from build123d import *

# Parameters (mm, degrees)
F0_W     = 72.5
F0_H     = 50
F1_DEPTH = 3
F2_R     = 5
F4_DEPTH = 8
F5_R     = 3
F7_DEPTH = 33
F8_R     = 2


with BuildPart() as f1:
    # F0 (on Top) → F1 (new body)
    with BuildSketch(Plane.XY):
        Rectangle(F0_W, F0_H)
    extrude(amount=F1_DEPTH)

    # F2
    f2_edges = [f1.edges().sort_by_distance(p)[0] for p in [
        (36.25, -25, 1.5),
        (-36.25, -25, 1.5),
    ]]
    fillet(f2_edges, radius=F2_R)

    # F3 (on face) → F4 (join)
    with BuildSketch(Plane(origin=(0, 25, 0), x_dir=(-1, 0, 0), z_dir=(0, 1, 0))):
        with BuildLine():
            Line((36.25, 3), (36.25, 8.712942712))
            ThreePointArc((36.25, 8.712942712), (0, 11.712942712), (-36.25, 8.712942712))
            Line((-36.25, 8.712942712), (-36.25, 3))
            Line((-36.25, 3), (36.25, 3))
        make_face()
    extrude(amount=-F4_DEPTH)

    # F5
    f5_edges = [f1.edges().sort_by_distance(p)[0] for p in [
        (36.25, 21, 8.712943),
        (-36.25, 21, 8.712943),
    ]]
    fillet(f5_edges, radius=F5_R)

    # F6 (on face) → F7 (join)
    with BuildSketch(Plane.XZ.offset(-17)):
        with BuildLine():
            Line((32.25, 3), (36.25, 3))
            Line((36.25, 3), (36.25, 6.1565184682))
            ThreePointArc((36.25, 6.1565184682), (35.527695785, 8.1089789443), (33.7085987261, 9.1212591328))
            ThreePointArc((33.7085987261, 9.1212591328), (32.9794838617, 9.2327934458), (32.25, 9.3418882854))
            Line((32.25, 9.3418882854), (32.25, 3))
        make_face()
    extrude(amount=F7_DEPTH)

    # F8
    f8_edges = [f1.edges().sort_by_distance(p)[0] for p in [
        (36.25, -16, 4.578259),
    ]]
    fillet(f8_edges, radius=F8_R)

    # F9: F1 across plane


with BuildPart() as f1_1:
    add(f1.part)
    add(f1.part.mirror(Plane.YZ))


solid = f1_1.part
Source: CAD feature listing. Evaluate the final solid. Frame: model axes, mm. A direction names the side the tool comes from. Round coordinates to 2 decimals unless told otherwise and drop trailing zeros. Write each loop counter-clockwise with the first axis right and the second up, starting at its lowest first coordinate (ties: lowest second). Pieces come first, ordered by that corner, then holes. Notation, with made-up numbers: (49, 53.5) - (77, 53.5) arc R14 ccw to (77, 79.5) - close; hole circle Ø11 at (-39.5, 53.25). An arc over 180 degrees is marked (long way). Use CSV: the item, a comma, the result in double quotes. Start each with the question number.
(1) Set-up query: faces 1 (the face through (35.68, -15.4, 4.6)), 2 (the face through (-32.25, 1, 6)), 3 (the face through (-34.82, -23.5, 1.52)), 4 (the face through (33, -16, 5)). Return all of +Z, -Z, +X, -X, +Y, -Y with unobstructed straight access to the full face (end or side cutting, diameter ignored); none if empty.
(2) Cut plane C-C, the plane y = -7.5. Return loops of the section in (x, z), and give its area (3 significant figures).
(3) Mould query, pull axis X, two halves, no side actions, for faces 5 (the face through (-35.68, -15.4, 4.6)), 6 (the face through (-33, -16, 5)), 7 (the face through (0, 17, 7)). Classes: pulls with the +X half, pulls with the -X half, needs draft (parallel to the pull), parting line crosses it, or undercut.
(4) Material intervals for probe 1 along Y at (x, z) = (11, 10); probe 2 along Z at (x, y) = (-15.5, 12.5); probe 3 along X at (y, z) = (-22.5, 2.5), sorted ascending. Write a range as [from, to].
(5) First-contact query: pin 1 Ø4 at (x, y) = (-27.5, -16.5) entering from +Z; pin 2 Ø2 at (x, z) = (-33, 5) entering from -Y; pin 3 Ø3 at (x, z) = (-7, 9.5) entering from -Y; pin 4 Ø6 at (x, y) = (-5.5, 9) entering from -Z. Flat tips, straight axial feed; report the tip coordinate or a pass-through.
(6) Cut plane A-A, the plane y = 18.5. Return loops of the section in (x, z).
(7) Cut plane B-B, the plane x = 20. Return loops of the section in (y, z), and give its area (3 significant figures).
Geometry says:
1,face 1,"+Z, +X, -Y"
1,face 2,"+Z, -Y"
1,face 3,"+Z, -Z, -X, -Y"
1,face 4,"+Z, +X, -X, -Y"
2,outline,"(-36.25, 0) - (36.25, 0) - (36.25, 6.16) arc R3 ccw to (33.71, 9.12) arc R220.51 ccw to (32.25, 9.34) - (32.25, 3) - (-32.25, 3) - (-32.25, 9.34) arc R220.51 ccw to (-33.71, 9.12) arc R3 ccw to (-36.25, 6.16) - close"
2,area,"263 mm²"
3,face 5,"pulls with the -X half"
3,face 6,"needs draft"
3,face 7,"undercut"
4,probe 1,"[17, 25]"
4,probe 2,"[0, 3]"
4,probe 3,"[-35.58, 35.58]"
5,pin 1,"z = 3"
5,pin 2,"y = -16"
5,pin 3,"y = 17"
5,pin 4,"z = 0"
6,outline,"(-36.25, 0) - (36.25, 0) - (36.25, 6.16) arc R3 ccw to (33.71, 9.12) arc R220.51 ccw to (-33.71, 9.12) arc R3 ccw to (-36.25, 6.16) - close"
7,outline,"(-25, 0) - (25, 0) - (25, 10.8) - (17, 10.8) - (17, 3) - (-25, 3) - close"
7,area,"212 mm²"
